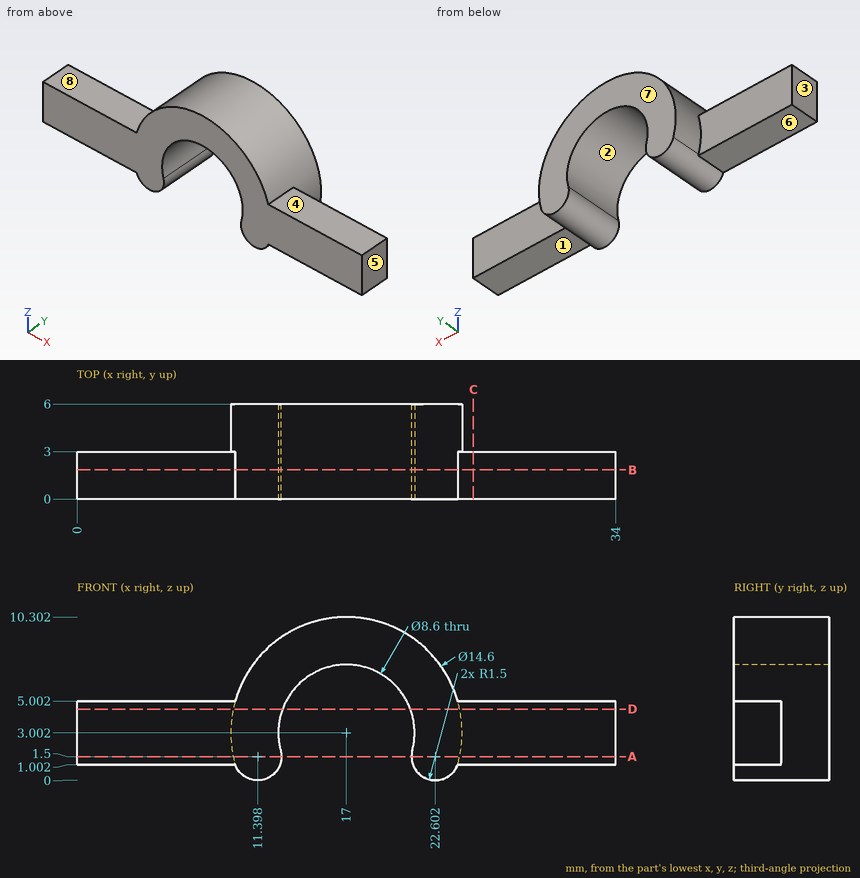
The drawing under review shows one solid part. Ordinate dimensions are in mm from its lowest x, y, z. A direction names the side the tool comes from. Coordinates: 2 decimals unless noted, no trailing zeros. Write each loop counter-clockwise with the first axis right and the second up, starting at its lowest first coordinate (ties: lowest second). Pieces come first, ordered by that corner, then holes.
1) Add section D-D (z = 4.5). Write out the cut boundary in (x, y) (1 decimal), plus the area to 3 significant figures.
2) To check wall thickness, follow L1, parallel to Z at x = 24.5, y = 0.9; L2, parallel to Y at x = 32, z = 1.25; L3, parallel to Z at x = 17, y = 3.9. State the ranges of each line that lie inside material, in increasing order.
3) Machinability: for the marked faces 4, 5, 6, 7 and 8, which of the approach directions +Z, -Z, +X, -X, +Y, -Y give a long, thin tool a straight path to every point of the face, cutting with its end or side? Answer none if there is none.
4) Add section B-B (y = 1.85). Write out the cut boundary in (x, z).
5) Mouldability with a two-part tool opening along Z and no side actions: class the marked faces 1, 2 and 3 as +Z half, -Z half, draft (parallel to the pull), parting line (faces both ways), or undercut.
6) Add section A-A (z = 1.5). Write out the cut boundary in (x, y).
7) Insertion check: pin 1 (4.5 mm diameter, centred on x = 3.5, z = 3, fed in from +Y); pin 2 (2.5 mm diameter, centred on x = 3.5, y = 1.5, fed in from -Z); pin 3 (1.5 mm diameter, centred on x = 3, y = 1.5, fed in from +Z). Each pin has a flat end and moves straight along its axis. Give the tip position at first contact, or say it passes through.
8) Add section C-C (x = 25). Write out the cut boundary in (y, z).
Check result:
1. outline: (0, 0) - (13, 0) - (13, 6) - (9.9, 6) - (9.9, 3) - (0, 3) - close; (21, 0) - (34, 0) - (34, 3) - (24.1, 3) - (24.1, 6) - (21, 6) - close
1. area: 96.5 mm2
2. L1: z = 1 to 5
2. L2: y = 0 to 3
2. L3: z = 7.3 to 10.3
3. face 4: +Z, +X, +Y, -Y
3. face 5: +Z, -Z, +X, +Y, -Y
3. face 6: -Z, -X, +Y, -Y
3. face 7: +Z, -Z, +X, -X, +Y
3. face 8: +Z, -X, +Y, -Y
4. outline: (0, 1) - (9.98, 1) arc R1.5 ccw to (12.85, 1.89) arc R4.3 cw (long way) to (21.15, 1.89) arc R1.5 ccw to (24.02, 1) - (34, 1) - (34, 5) - (24.02, 5) arc R7.3 ccw to (9.98, 5) - (0, 5) - close
5. face 1: -Z half
5. face 2: undercut
5. face 3: draft
6. outline: (0, 0) - (12.9, 0) - (12.9, 6) - (9.86, 6) - (9.86, 3) - (0, 3) - close; (21.1, 0) - (34, 0) - (34, 3) - (24.14, 3) - (24.14, 6) - (21.1, 6) - close
7. pin 1: stops at y = 3
7. pin 2: stops at z = 1
7. pin 3: stops at z = 5
8. outline: (0, 1) - (3, 1) - (3, 5) - (0, 5) - close
